Read the model definition and answer for the solid it produces. Units are mm, in the model's axes. Coordinates: 2 decimals unless noted, no trailing zeros. Loops run counter-clockwise (first coordinate to the right, second up) from the corner with the lowest first, then second, coordinate; pieces in that order, holes last. Notation, with made-up numbers: M 58,-40 L 63,-40 A12 cw 63,-27 Z; hole C 15.25,-22 d10. An arc over 180 degrees is marked long. Put each result on its own line as item: value.
from build123d import *

# Parameters (mm, degrees)
SKETCH1_W           = 101.6
SKETCH1_H           = 114.3
BOSS_EXTRUDE2_DEPTH = 6.35
SKETCH4_W           = 152.4
SKETCH4_H           = 152.4
SKETCH4_W_2         = 101.6
SKETCH4_H_2         = 114.3
BOSS_EXTRUDE4_DEPTH = 6.35
FILLET1_R           = 10
SKETCH5_R           = 3.175
CUT_EXTRUDE1_DEPTH  = 6.35


with BuildPart() as part:
    # Sketch1 → Boss-Extrude2 (new body)
    with BuildSketch(Plane(origin=(0, 0, 0), x_dir=(1, 0, 0), z_dir=(0, 1, 0))):
        Rectangle(SKETCH1_W, SKETCH1_H)
        with BuildLine():
            ThreePointArc((33.812535371, 35.527521223), (40.672478777, 33.812535371), (42.387464629, 40.672478777))
            Line((42.387464629, 40.672478777), (37.624964629, 48.609978777))
            ThreePointArc((37.624964629, 48.609978777), (30.765021223, 50.324964629), (29.050035371, 43.465021223))
            Line((29.050035371, 43.465021223), (33.812535371, 35.527521223))
        make_face(mode=Mode.SUBTRACT)
        with BuildLine():
            ThreePointArc((-33.812535371, -35.527521223), (-40.672478777, -33.812535371), (-42.387464629, -40.672478777))
            Line((-42.387464629, -40.672478777), (-37.624964629, -48.609978777))
            ThreePointArc((-37.624964629, -48.609978777), (-30.765021223, -50.324964629), (-29.050035371, -43.465021223))
            Line((-29.050035371, -43.465021223), (-33.812535371, -35.527521223))
        make_face(mode=Mode.SUBTRACT)
        with BuildLine():
            ThreePointArc((-33.812535371, 35.527521223), (-40.672478777, 33.812535371), (-42.387464629, 40.672478777))
            Line((-42.387464629, 40.672478777), (-37.624964629, 48.609978777))
            ThreePointArc((-37.624964629, 48.609978777), (-30.765021223, 50.324964629), (-29.050035371, 43.465021223))
            Line((-29.050035371, 43.465021223), (-33.812535371, 35.527521223))
        make_face(mode=Mode.SUBTRACT)
        with BuildLine():
            Line((29.050035371, -43.465021223), (33.812535371, -35.527521223))
            ThreePointArc((33.812535371, -35.527521223), (40.672478777, -33.812535371), (42.387464629, -40.672478777))
            Line((42.387464629, -40.672478777), (37.624964629, -48.609978777))
            ThreePointArc((37.624964629, -48.609978777), (30.765021223, -50.324964629), (29.050035371, -43.465021223))
        make_face(mode=Mode.SUBTRACT)
    extrude(amount=BOSS_EXTRUDE2_DEPTH)

    # Sketch4 → Boss-Extrude4 (add)
    with BuildSketch(Plane(origin=(0, 6.35, 0), x_dir=(1, 0, 0), z_dir=(0, 1, 0))):
        Rectangle(SKETCH4_W, SKETCH4_H)
        Rectangle(SKETCH4_W_2, SKETCH4_H_2, mode=Mode.SUBTRACT)
    extrude(amount=-BOSS_EXTRUDE4_DEPTH)

    # Fillet1
    fillet1_edges = [part.edges().sort_by_distance(p)[0] for p in [
        (76.2, 3.175, -76.2),
        (76.2, 3.175, 76.2),
        (-76.2, 3.175, 76.2),
        (-76.2, 3.175, -76.2),
    ]]
    fillet(fillet1_edges, radius=FILLET1_R)

    # Sketch5 → Cut-Extrude1 (cut)
    with BuildSketch(Plane(origin=(0, 6.35, 0), x_dir=(1, 0, 0), z_dir=(0, 1, 0))):
        with Locations((-25.4, 0)):
            Circle(SKETCH5_R)
        with Locations((-50.8, 0)):
            Circle(SKETCH5_R)
        with Locations((50.8, 0)):
            Circle(SKETCH5_R)
        with Locations((0, -25.4)):
            Circle(SKETCH5_R)
        with Locations((-63.5, -38.5)):
            Circle(SKETCH5_R)
        with Locations((-63.5, -63.5)):
            Circle(SKETCH5_R)
        with Locations((-38.1, -63.5)):
            Circle(SKETCH5_R)
        with Locations((38.1, -63.5)):
            Circle(SKETCH5_R)
        with Locations((63.5, -38.5)):
            Circle(SKETCH5_R)
        with Locations((63.5, -63.5)):
            Circle(SKETCH5_R)
        with Locations((0, -50.8)):
            Circle(SKETCH5_R)
        with Locations((0, 25.4)):
            Circle(SKETCH5_R)
        with Locations((-63.5, 38.5)):
            Circle(SKETCH5_R)
        with Locations((-38.1, 63.5)):
            Circle(SKETCH5_R)
        Circle(SKETCH5_R)
        with Locations((25.4, 0)):
            Circle(SKETCH5_R)
        with Locations((63.5, 63.5)):
            Circle(SKETCH5_R)
        with Locations((63.5, 38.5)):
            Circle(SKETCH5_R)
        with Locations((38.1, 63.5)):
            Circle(SKETCH5_R)
        with Locations((0, 50.8)):
            Circle(SKETCH5_R)
        with Locations((-63.5, 63.5)):
            Circle(SKETCH5_R)
    extrude(amount=-CUT_EXTRUDE1_DEPTH, mode=Mode.SUBTRACT)


solid = part.part
1) Find section A-A, the plane x = 0. Write down the section's boundary in (y, z) (3 decimals), plus the area to 3 significant figures.
Answer list:
outline: M 0,-76.2 L 6.35,-76.2 L 6.35,-53.975 L 0,-53.975 Z; M 0,-47.625 L 6.35,-47.625 L 6.35,-28.575 L 0,-28.575 Z; M 0,-22.225 L 6.35,-22.225 L 6.35,-3.175 L 0,-3.175 Z; M 0,3.175 L 6.35,3.175 L 6.35,22.225 L 0,22.225 Z; M 0,28.575 L 6.35,28.575 L 6.35,47.625 L 0,47.625 Z; M 0,53.975 L 6.35,53.975 L 6.35,76.2 L 0,76.2 Z
area: 766 mm^2
2) Straight lines are drawn through the part: line 1 (Z direction, x = 0, y = 3.75) (3 decimals); line 2 (X direction, y = 3.25, z = 63.5) (3 decimals); line 3 (Z direction, x = 63.5, y = 3) (3 decimals). For each, find the intervals that lie inside material, in ascending order. Write a range as [from, to].
Answer list:
line 1: z = [-76.2, -53.975], [-47.625, -28.575], [-22.225, -3.175], [3.175, 22.225], [28.575, 47.625], [53.975, 76.2]
line 2: x = [-76.2, -66.675], [-60.325, -41.275], [-34.925, 34.925], [41.275, 60.325], [66.675, 76.2]
line 3: z = [-76.2, -66.675], [-60.325, -41.675], [-35.325, 35.325], [41.675, 60.325], [66.675, 76.2]
3) Given pin 1 Ø5 at (x, z) = (0, 25.4) entering from +Y, flat-ended and moving along its own axis, determine where the tip first touches the part or whether it passes through.
Answer list:
pin 1: passes through
4) Find section B-B, the plane z = 63.5. Write down the section's boundary in (x, y) (3 decimals).
Answer list:
outline: M -76.2,0 L -66.675,0 L -66.675,6.35 L -76.2,6.35 Z; M -60.325,0 L -41.275,0 L -41.275,6.35 L -60.325,6.35 Z; M -34.925,0 L 34.925,0 L 34.925,6.35 L -34.925,6.35 Z; M 41.275,0 L 60.325,0 L 60.325,6.35 L 41.275,6.35 Z; M 66.675,0 L 76.2,0 L 76.2,6.35 L 66.675,6.35 Z
5) Find section D-D, the plane x = -25.4. Write down the section's boundary in (y, z) (3 decimals), plus the area to 3 significant figures.
Answer list:
outline: M 0,-76.2 L 6.35,-76.2 L 6.35,-3.175 L 0,-3.175 Z; M 0,3.175 L 6.35,3.175 L 6.35,76.2 L 0,76.2 Z
area: 927 mm^2
6) Determine the mould class of faces 1 (the flat face through (-1, 6.35, -18)), 2 (the cylindrical face through (73.19, 3.13, -73.35)), 3 (the cylindrical face through (-60.47, 3.22, -64.45)) for opening direction X: released by +X, released by -X, zero draft, split by the parting line, or undercut.
Answer list:
face 1: zero draft
face 2: released by +X
face 3: undercut
7) Find section C-C, the plane x = 63.5. Write down the section's boundary in (y, z) (3 decimals).
Answer list:
outline: M 0,-76.2 L 6.35,-76.2 L 6.35,-66.675 L 0,-66.675 Z; M 0,-60.325 L 6.35,-60.325 L 6.35,-41.675 L 0,-41.675 Z; M 0,-35.325 L 6.35,-35.325 L 6.35,35.325 L 0,35.325 Z; M 0,41.675 L 6.35,41.675 L 6.35,60.325 L 0,60.325 Z; M 0,66.675 L 6.35,66.675 L 6.35,76.2 L 0,76.2 Z
